The listing builds one solid part. Answer for the finished solid, in the listing's coordinates (mm). Face numbers are marked on the shaded views. A direction names the side the tool comes from. Coordinates: 2 decimals unless noted, no trailing zeros. Order: outer loops, then holes, each group sorted by start corner. A loop starts at its lowest first (then second) coordinate and runs counter-clockwise, first axis right, second up. Notation, with made-up numbers: (11.25, 65.25) - (69.25, 65.25) arc R20 cw to (69.25, 71.25) - close; hole circle Ø7 at (70, 51.5). An arc over 180 degrees is marked (long way). Use a Markdown table: item, result. Add a question column.
Item 1: The part is cut by section A-A, the plane z = -9.5. Give the vertices of the cut face in (x, y), then the cut area to 3 significant figures.
Item 2: The part is cut by section B-B, the plane y = -10. Give the vertices of the cut face in (x, z).
Item 3: Find the intervals of material crossed by line 1 along X through (y, z) = (-13.5, -18); line 2 along Y through (x, z) = (-7, -5); line 3 along X through (y, z) = (-3.75, 23), in increasing order.
Item 4: For the marked faces 4 and 5, determine the directions among +Z, -Z, +X, -X, +Y, -Y from which every point of the face is accessible in a straight line to the end or side of a thin tool.
Item 5: Flat-ended cylindrical pins translate along their axes: P1, Ø3, axis at x = -8, z = -8, coming from the -Y side; P2, Ø6.5, axis at y = 5, z = 4.5, coming from the -X side; P3, Ø2, axis at x = -15.64, z = -38.22, coming from the -Y side; P4, Ø2, axis at x = 14.5, z = -6.5, coming from the +Y side. Find the tip coordinate at first contact, or state that the pin passes through.
Item 6: The mould has two halves that part along X. Classify the marked faces 1, 2 and 3: released by +X, released by -X, zero draft, split by the parting line, or undercut.
Item 7: The part is cut by section C-C, the plane y = 1.5. Give the vertices of the cut face in (x, z).
from build123d import *

# Parameters (mm, degrees)
SKETCH001_W   = 38.64
SKETCH001_H   = 68.64
PAD001_DEPTH  = 20
THICKNESS_T   = -4
FILLET002_R   = 1
PAD006_DEPTH  = 16
SKETCH013_R   = 1.2
HOLE002_DEPTH = 25
FILLET004_R   = 1
SKETCH018_W   = 12
SKETCH018_H   = 40
PAD008_DEPTH  = 4
SKETCH019_W   = 20
SKETCH019_H   = 40
PAD009_DEPTH  = 4
SKETCH020_W   = 20
SKETCH020_H   = 8
PAD010_DEPTH  = 4


with BuildPart() as part:
    # Sketch001 → Pad001 (new body)
    with BuildSketch(Plane.XZ):
        with Locations((-0.32, -7.9)):
            Rectangle(SKETCH001_W, SKETCH001_H)
    extrude(amount=PAD001_DEPTH)

    # Thickness
    thickness_openings = [part.faces().sort_by_distance(p)[0] for p in [
        (-0.32, -20, -7.9),
    ]]
    offset(amount=THICKNESS_T, openings=thickness_openings)

    # Fillet002
    fillet002_edges = [part.edges().sort_by_distance(p)[0] for p in [
        (-19.64, -10, 26.42),
        (19, -10, 26.42),
        (19, -10, -42.22),
        (-19.64, -10, -42.22),
        (-19.64, 0, -7.9),
        (-0.32, 0, -42.22),
        (19, 0, -7.9),
        (-0.32, 0, 26.42),
    ]]
    fillet(fillet002_edges, radius=FILLET002_R)

    # Sketch012 (on Face23 of Fillet002) → Pad006 (join)
    with BuildSketch(Plane.XZ.offset(4)):
        with BuildLine():
            ThreePointArc((-11.32, 22.42), (-14.374701, 21.154701), (-15.64, 18.1))
            Line((-15.64, 22.42), (-15.64, 18.1))
            Line((-11.32, 22.42), (-15.64, 22.42))
        make_face()
        with BuildLine():
            ThreePointArc((15, 18.1), (13.734701, 21.154701), (10.68, 22.42))
            Line((10.68, 22.42), (15, 22.42))
            Line((15, 22.42), (15, 18.1))
        make_face()
        with BuildLine():
            ThreePointArc((10.68, -38.22), (13.734701, -36.954701), (15, -33.9))
            Line((15, -38.22), (15, -33.9))
            Line((10.68, -38.22), (15, -38.22))
        make_face()
        with BuildLine():
            Line((-15.64, -38.22), (-15.64, -33.9))
            ThreePointArc((-15.64, -33.9), (-14.374701, -36.954701), (-11.32, -38.22))
            Line((-11.32, -38.22), (-15.64, -38.22))
        make_face()
    extrude(amount=PAD006_DEPTH)

    # Sketch013 (on Face12 of Pad006) → Hole002 (cut)
    with BuildSketch(Plane(origin=(0, 0, 0), x_dir=(-1, 0, 0), z_dir=(0, 1, 0))):
        with Locations((-15, 22.42)):
            Circle(SKETCH013_R)
        with Locations((15.64, 22.42)):
            Circle(SKETCH013_R)
        with Locations((-15, -38.22)):
            Circle(SKETCH013_R)
        with Locations((15.64, -38.22)):
            Circle(SKETCH013_R)
    extrude(amount=-HOLE002_DEPTH, mode=Mode.SUBTRACT)

    # Fillet004
    fillet004_edges = [part.edges().sort_by_distance(p)[0] for p in [
        (-16.84, 0, 22.42),
        (13.8, 0, 22.42),
        (13.8, 0, -38.22),
        (-16.84, 0, -38.22),
    ]]
    fillet(fillet004_edges, radius=FILLET004_R)

    # Sketch018 (on Face4 of Fillet004) → Pad008 (join)
    with BuildSketch(Plane(origin=(0, 0, 0), x_dir=(-1, 0, 0), z_dir=(0, 1, 0))):
        with Locations((0.32, -7.9)):
            Rectangle(SKETCH018_W, SKETCH018_H)
    extrude(amount=PAD008_DEPTH)

    # Sketch019 (on Face40 of Pad008) → Pad009 (join)
    with BuildSketch(Plane(origin=(0, 4, 0), x_dir=(-1, 0, 0), z_dir=(0, 1, 0))):
        with Locations((0.32, -7.9)):
            Rectangle(SKETCH019_W, SKETCH019_H)
    extrude(amount=PAD009_DEPTH)

    # Sketch020 (on Face44 of Pad009) → Pad010 (join)
    with BuildSketch(Plane.XY.offset(12.1)):
        with Locations((-0.32, 4)):
            Rectangle(SKETCH020_W, SKETCH020_H)
    extrude(amount=PAD010_DEPTH)


solid = part.part
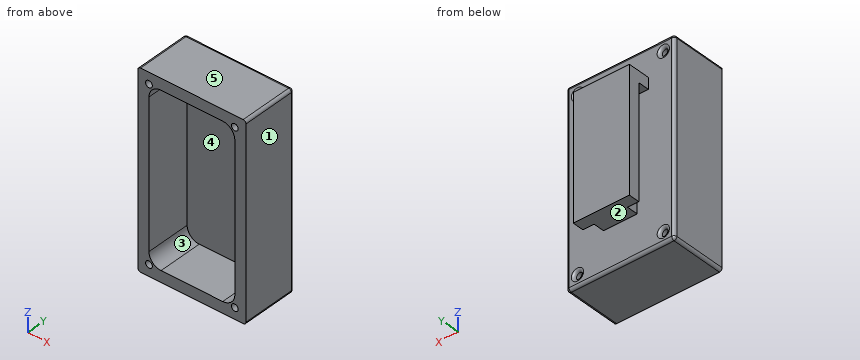
Solution:
| question | item | result |
|---|---|---|
| 1 | outline | (-19.64, -20) - (-15.64, -20) - (-15.64, -4) - (15, -4) - (15, -20) - (19, -20) - (19, -1) arc R1 ccw to (18, 0) - (5.68, 0) - (5.68, 4) - (9.68, 4) - (9.68, 8) - (-10.32, 8) - (-10.32, 4) - (-6.32, 4) - (-6.32, 0) - (-18.64, 0) arc R1 ccw to (-19.64, -1) - close |
| 1 | area | 410 mm2 |
| 2 | outline | (-19.64, -41.22) arc R1 ccw to (-18.64, -42.22) - (18, -42.22) arc R1 ccw to (19, -41.22) - (19, 25.42) arc R1 ccw to (18, 26.42) - (-18.64, 26.42) arc R1 ccw to (-19.64, 25.42) - close; hole circle Ø2.4 at (-15.64, -38.22); hole circle Ø2.4 at (-15.64, 22.42); hole (-15.64, -33.9) arc R4.32 ccw to (-11.32, -38.22) - (10.68, -38.22) arc R4.32 ccw to (15, -33.9) - (15, 18.1) arc R4.32 ccw to (10.68, 22.42) - (-11.32, 22.42) arc R4.32 ccw to (-15.64, 18.1) - close; hole circle Ø2.4 at (15, -38.22); hole circle Ø2.4 at (15, 22.42) |
| 3 | line 1 | x = -19.64 to -15.64, 15 to 19 |
| 3 | line 2 | y = -4 to 0, 4 to 8 |
| 3 | line 3 | x = -19.64 to -16.69, -14.59 to 13.95, 16.05 to 19 |
| 4 | face 4 | -Y |
| 4 | face 5 | +Z, +X, -X, +Y, -Y |
| 5 | P1 | stops at y = -4 |
| 5 | P2 | stops at x = -10.32 |
| 5 | P3 | passes through |
| 5 | P4 | stops at y = 0 |
| 6 | face 1 | released by +X |
| 6 | face 2 | zero draft |
| 6 | face 3 | undercut |
| 7 | outline | (-10.32, 12.1) - (-6.32, 12.1) - (-6.32, -27.9) - (5.68, -27.9) - (5.68, 12.1) - (9.68, 12.1) - (9.68, 16.1) - (-10.32, 16.1) - close |
